Here's how the part is built. I have some questions about the finished solid (model axes, mm). A direction names the side the tool comes from. Give positions to 0.01 mm unless a question says otherwise; leave off trailing zeros. Loops run counter-clockwise (first coordinate to the right, second up) from the corner with the lowest first, then second, coordinate; pieces in that order, holes last. Notation, with made-up numbers: M 81.25,58.25 L 97.25,58.25 A29 ccw 97.25,97.25 Z; hole C 70,58 d10. An arc over 180 degrees is marked long. Write item = value, one per line. Start each with the question number.
```python
from build123d import *

# Parameters (mm, degrees)
SKETCH_1_R          = 2
EXTRUDE_1_DEPTH     = 5
SKETCH_3_R          = 12.5
SKETCH_3_R_2        = 4
EXTRUDE_2_DEPTH     = 13
SKETCH_5_R          = 4
CUT_EXTRUDE_1_DEPTH = 26.039562279


with BuildPart() as part:
    # 草图1 → 凸台-拉伸1 (new body)
    with BuildSketch(Plane.XY):
        with BuildLine():
            Line((-12.459935794, -14.736328125), (12.459935794, -14.736328125))
            ThreePointArc((12.459935794, -14.736328125), (13.788582233, -13.524910358), (15, -12.196263919))
            Line((15, -12.196263919), (15, 12.723607669))
            ThreePointArc((15, 12.723607669), (13.788582233, 14.052254108), (12.459935794, 15.263671875))
            Line((12.459935794, 15.263671875), (-12.459935794, 15.263671875))
            ThreePointArc((-12.459935794, 15.263671875), (-13.788582233, 14.052254108), (-15, 12.723607669))
            Line((-15, 12.723607669), (-15, -12.196263919))
            ThreePointArc((-15, -12.196263919), (-13.788582233, -13.524910358), (-12.459935794, -14.736328125))
        make_face()
        with Locations((-11.347647071, 11.611318946)):
            Circle(SKETCH_1_R, mode=Mode.SUBTRACT)
        with Locations((11.313708499, 11.577380374)):
            Circle(SKETCH_1_R, mode=Mode.SUBTRACT)
        with Locations((11.313708499, -11.050036624)):
            Circle(SKETCH_1_R, mode=Mode.SUBTRACT)
        with Locations((-11.313708499, -11.050036624)):
            Circle(SKETCH_1_R, mode=Mode.SUBTRACT)
    extrude(amount=EXTRUDE_1_DEPTH)

    # 草图3 → 凸台-拉伸2 (add)
    with BuildSketch(Plane.XY.offset(5)):
        with Locations(Location((0, 0, 0), (0, 0, 180))):
            Circle(SKETCH_3_R)
        with Locations(Location((0, 0, 0), (0, 0, 180))):
            Circle(SKETCH_3_R_2, mode=Mode.SUBTRACT)
    extrude(amount=EXTRUDE_2_DEPTH)

    # 草图5 → 切除-拉伸1 (cut, through all)
    with BuildSketch(Plane.XY.offset(5)):
        with Locations(Location((0, 0, 0), (0, 0, 180))):
            Circle(SKETCH_5_R)
    extrude(amount=-CUT_EXTRUDE_1_DEPTH, mode=Mode.SUBTRACT)


solid = part.part
```
Q1. If we section it at C-C, the plane z = 4: List the corners of the cut face in (x, y) for me.
Q2. On a 3-axis mill with a long thin cutter (end or side, diameter ignored), from which of +Z, -Z, +X, -X, +Y, -Y can I reach the whole of each face in a straight line? I mean faces 1 (the cylindrical face through (-11.923, -3.755, 11.409)), 2 (the cylindrical face through (13.771, -13.543, 2.465)). Say none if no direction works.
Q3. If I drill on line 1 along X through (y, z) = (13, 1.5); line 2 along X through (y, z) = (-10, 3.5); line 3 along Y through (x, z) = (0, 1.85), over which ranges is the centre line in solid material (lowest first)?
Q4. If we section it at B-B, the plane y = 0: List the corners of the cut face in (x, z) for me.
Q5. We'd pull the mould along Y, two halves only. Please class faces 3 (the flat face through (0, 15.264, 2)), 4 (the flat face through (15, 0, 2)), 5 (the flat face through (0, -14.736, 2)), 6 (the cylindrical face through (-12.79, -9.7, 2.46)): pulls with the +Y half, pulls with the -Y half, needs draft (parallel to the pull), parting line crosses it, or undercut.
Q6. If we section it at A-A, the plane x = 0: List the corners of the cut face in (y, z) for me.
Q7. If we section it at D-D, the plane y = 7.5: List the corners of the cut face in (x, z) for me, then the cut area to 3 significant figures.
Q8. Will these pins go through, and if not, where does the flat tip stop? pin 1 (8 mm diameter, centred on x = 9, z = 12, fed in from +Y); pin 2 (2.5 mm diameter, centred on x = 11.31, y = -11.05, fed in from -Z); pin 3 (4.5 mm diameter, centred on x = -11.31, y = -11.05, fed in from +Z); pin 4 (3 mm diameter, centred on y = -7, z = 16, fed in from +X) (3 decimals).
Resolved:
q1.outline = M -15,-12.2 A19.5 ccw -12.46,-14.74 L 12.46,-14.74 A19.5 ccw 15,-12.2 L 15,12.72 A19.5 ccw 12.46,15.26 L -12.46,15.26 A19.5 ccw -15,12.72 Z; hole C -11.35,11.61 d4; hole C -11.31,-11.05 d4; hole C 0,0 d8; hole C 11.31,-11.05 d4; hole C 11.31,11.58 d4
q2.face_1 = +Z
q2.face_2 = +Z, -Z, +X, -Y
q3.line_1 = -14.77 to -12.79, -9.91 to 9.91, 12.72 to 14.77
q3.line_2 = -15 to -13.02, -9.61 to 9.61, 13.02 to 15
q3.line_3 = -14.74 to -4, 4 to 15.26
q4.outline = M -15,0 L -4,0 L -4,18 L -12.5,18 L -12.5,5 L -15,5 Z; M 4,0 L 15,0 L 15,5 L 12.5,5 L 12.5,18 L 4,18 Z
q5.face_3 = pulls with the +Y half
q5.face_4 = needs draft
q5.face_5 = pulls with the -Y half
q5.face_6 = undercut
q6.outline = M -14.74,0 L -4,0 L -4,18 L -12.5,18 L -12.5,5 L -14.74,5 Z; M 4,0 L 15.26,0 L 15.26,5 L 12.5,5 L 12.5,18 L 4,18 Z
q7.outline = M -15,0 L 15,0 L 15,5 L 10,5 L 10,18 L -10,18 L -10,5 L -15,5 Z
q7.area = 410 mm²
q8.pin_1 = 11.46
q8.pin_2 = through
q8.pin_3 = 5
q8.pin_4 = 11.225
